from build123d import *

# Parameters (mm, degrees)
SKETCH1_R           = 1.2
BOSS_EXTRUDE1_DEPTH = 2.5
SKETCH2_W           = 32.3
SKETCH2_H           = 15
BOSS_EXTRUDE2_DEPTH = 15.7


with BuildPart() as part:
    # Sketch1 → Boss-Extrude1 (new body)
    with BuildSketch(Plane.XY):
        Polygon((0, 0), (0, 27.5), (4.8, 27.5), (4.8, 15), (27.5, 15), (27.5, 27.5), (32.3, 27.5), (32.3, 0), align=None)
        with Locations((2.25, 21.25)):
            Circle(SKETCH1_R, mode=Mode.SUBTRACT)
        with Locations((30.05, 21.25)):
            Circle(SKETCH1_R, mode=Mode.SUBTRACT)
    extrude(amount=BOSS_EXTRUDE1_DEPTH)

    # Sketch2 → Boss-Extrude2 (add)
    with BuildSketch(Plane.XY.offset(2.5)):
        with Locations((16.15, 7.5)):
            Rectangle(SKETCH2_W, SKETCH2_H)
    extrude(amount=BOSS_EXTRUDE2_DEPTH)


solid = part.part
For this review, take the finished solid that the model builds, in its own axes (mm). A direction names the side the tool comes from. Give positions to 0.01 mm unless a question says otherwise; leave off trailing zeros. Write each loop counter-clockwise with the first axis right and the second up, starting at its lowest first coordinate (ties: lowest second). Pieces come first, ordered by that corner, then holes. Notation, with made-up numbers: (84, -24) -> (98, -24) arc R18 ccw to (98, -16) -> close; hole circle Ø6 at (36.25, 50.25). An arc over 180 degrees is marked (long way). Use CSV: the item, a comma, the result in double quotes.
Q1. Take a section at B-B, the plane x = 2.25. Write out the cut boundary in (y, z).
Conclusion:
outline,"(0, 0) -> (20.05, 0) -> (20.05, 2.5) -> (15, 2.5) -> (15, 18.2) -> (0, 18.2) -> close; (22.45, 0) -> (27.5, 0) -> (27.5, 2.5) -> (22.45, 2.5) -> close"
Q2. Tool access review of faces 4 (the face through (4.8, 21, 1)), 5 (the face through (4, 21, 2.5)), 6 (the face through (2.804, 20.185, 1.232)): name each direction out of +Z, -Z, +X, -X, +Y, -Y from which nothing blocks a thin tool from reaching the whole face with its end or side.
Conclusion:
face 4,"+Z, -Z, +Y"
face 5,"+Z, +X, -X, +Y"
face 6,"+Z, -Z"
Q3. Take a section at C-C, the plane y = 18.5. Write out the cut boundary in (x, z), then the cut area to 3 significant figures.
Conclusion:
outline,"(0, 0) -> (4.8, 0) -> (4.8, 2.5) -> (0, 2.5) -> close; (27.5, 0) -> (32.3, 0) -> (32.3, 2.5) -> (27.5, 2.5) -> close"
area,"24.0 mm2"
Q4. Take a section at D-D, the plane x = 12.5. Write out the cut boundary in (y, z), then the cut area to 3 significant figures.
Conclusion:
outline,"(0, 0) -> (15, 0) -> (15, 18.2) -> (0, 18.2) -> close"
area,"273 mm2"
Q5. To check wall thickness, follow probe 1 along Y at (x, z) = (2.25, 0.95); probe 2 along Y at (x, z) = (3, 7). State the ranges of each line that lie inside material, in increasing order. Write a range as [from, to].
Conclusion:
probe 1,"[0, 20.05], [22.45, 27.5]"
probe 2,"[0, 15]"
Q6. Take a section at A-A, the plane y = 21.25. Write out the cut boundary in (x, z), then the cut area to 3 significant figures.
Conclusion:
outline,"(0, 0) -> (1.05, 0) -> (1.05, 2.5) -> (0, 2.5) -> close; (3.45, 0) -> (4.8, 0) -> (4.8, 2.5) -> (3.45, 2.5) -> close; (27.5, 0) -> (28.85, 0) -> (28.85, 2.5) -> (27.5, 2.5) -> close; (31.25, 0) -> (32.3, 0) -> (32.3, 2.5) -> (31.25, 2.5) -> close"
area,"12.0 mm2"
Q7. For P1, Ø2.5, axis at x = 30.5, y = 20, coming from the +Z side; P2, Ø9, axis at x = 24, z = 5.5, coming from the +Y side; P3, Ø1.4, axis at x = 30.05, y = 21.25, coming from the -Z side, all flat-tipped, find the tip position at first contact; note any pin that passes through.
Conclusion:
P1,"z = 2.5"
P2,"y = 15"
P3,"through"
Q8. Mouldability with a two-part tool opening along Y and no side actions: class faces 1 (the face through (29.1, 20.52, 1.23)), 2 (the face through (29.9, 19.9, 2.5)), 3 (the face through (30, 27.5, 1)) as pulls with the +Y half, pulls with the -Y half, needs draft (parallel to the pull), parting line crosses it, or undercut.
Conclusion:
face 1,"undercut"
face 2,"needs draft"
face 3,"pulls with the +Y half"
